```python
from build123d import *

# Parameters (mm, degrees)
SKETCH2_R           = 2.25
BOSS_EXTRUDE1_DEPTH = 12.7
FILLET1_R           = 6.35
FILLET2_R           = 2
CUT_EXTRUDE2_START  = 12.7
SKETCH3_R           = 4.7625
SKETCH3_R_2         = 2.25
CUT_EXTRUDE2_DEPTH  = 6.35
SKETCH3_3_R         = 2.25
BOSS_EXTRUDE2_DEPTH = 12.7
FILLET3_R           = 6.35
CUT_EXTRUDE3_REACH  = 181.366
SKETCH4_R           = 2.25
CUT_EXTRUDE4_START  = 12.7
SKETCH3_4_R         = 2.25
CUT_EXTRUDE4_DEPTH  = 182.75835677
FILLET4_R           = 12.7


with BuildPart() as part:
    # Sketch2 → Boss-Extrude1 (new body)
    with BuildSketch(Plane(origin=(0, 0, 0), x_dir=(0, 0, -1), z_dir=(1, 0, 0))):
        Polygon((-41.425693669, -95.25), (142.682929389, -95.25), (51.328891162, 101.953428549), (-5.433161507, 3.638669384), align=None)
        Circle(SKETCH2_R, mode=Mode.SUBTRACT)
        with Locations((50.8, 87.988181024)):
            Circle(SKETCH2_R, mode=Mode.SUBTRACT)
        with Locations((-32.356953826, -88.9)):
            Circle(SKETCH2_R, mode=Mode.SUBTRACT)
        with Locations((132.743046174, -88.9)):
            Circle(SKETCH2_R, mode=Mode.SUBTRACT)
        with Locations((5.743046174, -88.9)):
            Circle(SKETCH2_R, mode=Mode.SUBTRACT)
        with Locations((94.643046174, -88.9)):
            Circle(SKETCH2_R, mode=Mode.SUBTRACT)
        Polygon((-23.288213983, -82.55), (3.196675109, -9.783365262), (111.849821959, -82.55), align=None, mode=Mode.SUBTRACT)
        Polygon((8.615197161, 1.87277804), (117.46426423, -71.025067394), (50.271108838, 74.0229335), align=None, mode=Mode.SUBTRACT)
    extrude(amount=BOSS_EXTRUDE1_DEPTH)

    # Fillet1
    fillet1_edges = [part.edges().sort_by_distance(p)[0] for p in [
        (6.35, 3.638669384, 5.433161507),
        (6.35, 101.953428549, -51.328891162),
        (6.35, -95.25, -142.682929389),
        (6.35, -95.25, 41.425693669),
    ]]
    fillet(fillet1_edges, radius=FILLET1_R)

    # Fillet2
    fillet2_edges = [part.edges().sort_by_distance(p)[0] for p in [
        (6.35, -82.55, 23.288213983),
        (6.35, -82.55, -111.849821959),
        (6.35, -9.783365262, -3.196675109),
        (6.35, 74.0229335, -50.271108838),
        (6.35, 1.87277804, -8.615197161),
        (6.35, -71.025067394, -117.46426423),
    ]]
    fillet(fillet2_edges, radius=FILLET2_R)

    # Sketch3 → Cut-Extrude2 (cut)
    with BuildSketch(Plane(origin=(0, 0, 0), x_dir=(0, 0, -1), z_dir=(1, 0, 0)).offset(CUT_EXTRUDE2_START)):
        with Locations((47.484762838, -31.801254664)):
            Circle(SKETCH3_R)
        with Locations((47.484762838, -31.801254664)):
            Circle(SKETCH3_R_2, mode=Mode.SUBTRACT)
    extrude(amount=-CUT_EXTRUDE2_DEPTH, mode=Mode.SUBTRACT)

    # Sketch3<3> → Boss-Extrude2 (add)
    # profile 1 of 2: a face of its own
    with BuildSketch(Plane(origin=(0, 0, 0), x_dir=(0, 0, -1), z_dir=(1, 0, 0))):
        Polygon((56.34256904, -7.163442885), (45.742150819, -22.991697164), (77.398659377, -44.192533607), (87.999077599, -28.364279328), align=None)
        with Locations((79.189520098, -30.106891347)):
            Circle(SKETCH3_3_R, mode=Mode.SUBTRACT)
        with Locations((58.085181059, -15.973000385)):
            Circle(SKETCH3_3_R, mode=Mode.SUBTRACT)
    # profile 2 of 2: a face of its own
    with BuildSketch(Plane(origin=(0, 0, 0), x_dir=(0, 0, -1), z_dir=(1, 0, 0))):
        Polygon((59.731295675, -70.572957406), (70.331713896, -54.744703127), (38.675205338, -33.543866684), (28.074787116, -49.372120963), align=None)
        with Locations((57.988683656, -61.763399906)):
            Circle(SKETCH3_3_R, mode=Mode.SUBTRACT)
        with Locations((36.884344616, -47.629508944)):
            Circle(SKETCH3_3_R, mode=Mode.SUBTRACT)
    extrude(amount=BOSS_EXTRUDE2_DEPTH)

    # Fillet3
    fillet3_edges = [part.edges().sort_by_distance(p)[0] for p in [
        (6.35, -28.364279328, -87.999077599),
        (6.35, -7.163442885, -56.34256904),
        (6.35, -49.372120963, -28.074787116),
        (6.35, -70.572957406, -59.731295675),
    ]]
    fillet(fillet3_edges, radius=FILLET3_R)

    # Sketch4 → Cut-Extrude3 (cut, up to next)
    with BuildSketch(Plane(origin=(0, 37.590233469, -81.144994396), x_dir=(-1, 0, 0), z_dir=(0, 0.4203363295122345, -0.9073683761803595)), mode=Mode.PRIVATE) as cut_extrude3_sk1:
        with Locations(Location((-6.35, 20.598120023, 0), (0, 0, 90))):
            Circle(SKETCH4_R)
    cut_extrude3_tool1 = extrude(cut_extrude3_sk1.sketch, amount=-CUT_EXTRUDE3_REACH, mode=Mode.PRIVATE) & part.part
    # Sketch4 → Cut-Extrude3 (cut, up to next)
    with BuildSketch(Plane(origin=(0, 37.590233469, -81.144994396), x_dir=(-1, 0, 0), z_dir=(0, 0.4203363295122345, -0.9073683761803595)), mode=Mode.PRIVATE) as cut_extrude3_sk2:
        with Locations(Location((-6.35, 33.298120023, 0), (0, 0, 90))):
            Circle(SKETCH4_R)
    cut_extrude3_tool2 = extrude(cut_extrude3_sk2.sketch, amount=-CUT_EXTRUDE3_REACH, mode=Mode.PRIVATE) & part.part
    add(cut_extrude3_tool1.solids().sort_by_distance((6.35, 56.280316, -72.486856))[0], mode=Mode.SUBTRACT)
    add(cut_extrude3_tool2.solids().sort_by_distance((6.35, 67.803895, -67.148585))[0], mode=Mode.SUBTRACT)

    # Sketch3<4> → Cut-Extrude4 (cut, through all)
    with BuildSketch(Plane(origin=(0, 0, 0), x_dir=(0, 0, -1), z_dir=(1, 0, 0)).offset(CUT_EXTRUDE4_START)):
        with Locations((47.484762838, -31.801254664)):
            Circle(SKETCH3_4_R)
    extrude(amount=-CUT_EXTRUDE4_DEPTH, mode=Mode.SUBTRACT)

    # Fillet4
    fillet4_edges = [part.edges().sort_by_distance(p)[0] for p in [
        (6.35, -44.192533607, -77.398659377),
        (6.35, -54.744703127, -70.331713896),
        (6.35, -22.991697164, -45.742150819),
        (6.35, -33.543866684, -38.675205338),
    ]]
    fillet(fillet4_edges, radius=FILLET4_R - 0.0001)  # a hair under: the kernel refuses the full size


solid = part.part
```
Work out the finished part from the listing and answer in its coordinate system (mm). A direction names the side the tool comes from. Coordinates: 2 decimals unless noted, no trailing zeros. Order: outer loops, then holes, each group sorted by start corner. A loop starts at its lowest first (then second) coordinate and runs counter-clockwise, first axis right, second up. Notation, with made-up numbers: M 26,68 L 63,68 A20 cw 63,94 Z; hole C -1.5,-26 d9. An arc over 180 degrees is marked long. Use CSV: the item, a comma, the result in double quotes.
1) Section A-A on y = -88.9 is taken. Write down the section's boundary in (x, z), plus the area to 3 significant figures.
Worked out:
outline,"M 0,-139.09 L 12.7,-139.09 L 12.7,-134.99 L 0,-134.99 Z; M 0,-130.49 L 12.7,-130.49 L 12.7,-96.89 L 0,-96.89 Z; M 0,-92.39 L 12.7,-92.39 L 12.7,-7.99 L 0,-7.99 Z; M 0,-3.49 L 12.7,-3.49 L 12.7,30.11 L 0,30.11 Z; M 0,34.61 L 12.7,34.61 L 12.7,38.71 L 0,38.71 Z"
area,"2,030 mm^2"
2) For faces 4 (the face through (9.569, -31.592, -42.727)), 5 (the face through (6.261, 2.04, -83.617)), 6 (the face through (0, -28, -56)), determine the directions among +Z, -Z, +X, -X, +Y, -Y from which every point of the face is accessible in a straight line to the end or side of a thin tool.
Worked out:
face 4,"+X"
face 5,"+X, -X"
face 6,"+Z, -Z, -X, +Y, -Y"
3) Section D-D on z = 25 is taken. Write down the section's boundary in (x, y), plus the area to 3 significant figures.
Worked out:
outline,"M 0,-95.25 L 12.7,-95.25 L 12.7,-50.12 L 0,-50.12 Z"
area,"573 mm^2"
4) Flat-ended cylindrical pins translate along their axes: pin 1 Ø6 at (y, z) = (-47.63, -36.88) entering from -X; pin 2 Ø1.5 at (x, z) = (9.5, -66.5) entering from +Y; pin 3 Ø3.5 at (y, z) = (-88.9, -5.74) entering from -X; pin 4 Ø5 at (x, y) = (7, -76) entering from +Z. Find the tip coordinate at first contact, or state that the pin passes through.
Worked out:
pin 1,"stops at x = 0"
pin 2,"stops at y = 70.82"
pin 3,"passes through"
pin 4,"stops at z = 35.33"
5) Determine the mould class of faces 1 (the face through (6.44, -92.61, 37.51)), 2 (the face through (7.026, 55.596, -65.904)), 3 (the face through (6.44, -92.39, -138.05)) for opening direction Z: released by +Z, released by -Z, zero draft, split by the parting line, or undercut.
Worked out:
face 1,"released by +Z"
face 2,"undercut"
face 3,"released by -Z"
6) Section B-B on y = 16.5 is taken. Write down the section's boundary in (x, z) (3 decimals).
Worked out:
outline,"M 0,-90.915 L 12.7,-90.915 L 12.7,-76.918 L 0,-76.918 Z; M 0,-17.06 L 12.7,-17.06 L 12.7,-1.992 L 0,-1.992 Z"
7) Consider line 1 (Y direction, x = 7.5, z = -25.5); line 2 (Y direction, x = 0.5, z = -99); line 3 (Z direction, x = 5.75, y = -1.5). Determine where each line is inside the solid, lowest interval first. Write a range as [from, to].
Worked out:
line 1,"y = [-95.25, -82.55], [-24.72, -9.44], [31.12, 57.22]"
line 2,"y = [-95.25, -82.55], [-73.94, -58.66], [-31.17, -0.95]"
line 3,"z = [-99.25, -85.26], [-13.65, -1.68], [1.68, 7.3]"
8) Section C-C on z = 0 is taken. Write down the section's boundary in (x, y), plus the area to 3 significant figures.
Worked out:
outline,"M 0,-95.25 L 12.7,-95.25 L 12.7,-82.55 L 0,-82.55 Z; M 0,-18.57 L 12.7,-18.57 L 12.7,-2.25 L 0,-2.25 Z; M 0,2.25 L 12.7,2.25 L 12.7,13.05 L 0,13.05 Z"
area,"506 mm^2"
